Solid Edge part; units mm, degrees
sketch "Sketch1" plane through (0, 0, 0) normal (0, -1, 0) x (1, 0, 0)
  line L0 (22.5, 0) -> (27.5, 0)
  line L1 (27.5, 0) -> (27.5, 5)
  line L2 (27.5, 5) -> (25.5, 5)
  line L3 (25.5, 5) -> (25.5, 10.1495)
  arc A0 (10, 12.9032) -> (25.5, 10.1495) centre (10, -32.0968) cw
  line L4 (0, 12.9032) -> (10, 12.9032)
  line L5 (0, 9.9032) -> (0, 12.9032)
  line L6 (0, 9.9032) -> (10, 9.9032)
  arc A1 (10, 9.9032) -> (22.5, 8) centre (10, -32.0968) cw
  line L7 (22.5, 8) -> (22.5, 0)
  dimension "D1" = 27.5
  dimension "D2" = 27.5
  dimension "D3" = 22.5
revolve "RevolvedProtrusion1" add sketch "Sketch1" angle 360 about axis through (0, 0, 0) along (0, 0, 1)
properties material "Steel"
Here's how the part is built. I have some questions about the finished solid (model axes, mm). A direction names the side the tool comes from. Coordinates: 2 decimals unless noted, no trailing zeros. Order: outer loops, then holes, each group sorted by start corner. A loop starts at its lowest first (then second) coordinate and runs counter-clockwise, first axis right, second up. Notation, with made-up numbers: (81, -37) - (136, -37) arc R11 cw to (136, -19) - close; hole circle Ø1 at (85.25, 43). An arc over 180 degrees is marked (long way). One line per question, with ' | ' between items. Start each with the question number.
1. Which directions (+Z, -Z, +X, -X, +Y, -Y) give clear straight access to the entire face, cutting with the end or side of a thin tool? Please do faces 1 (the flat face through (-23, 0, 0)), 2 (the flat face through (0, 0, 9.903)).
2. I'm going to push flat-ended pins straight in: pin 1 Ø3 at (y, z) = (-16.5, 1.5) entering from +X; pin 2 Ø2 at (x, y) = (21.5, 21.5) entering from +Z; pin 3 Ø16 at (x, y) = (-5, -1.5) entering from -Z; pin 4 Ø2 at (y, z) = (-14.5, 7) entering from -X. Where does each tip first touch, or does it pass through?
3. Please list where these lines run through material, in increasing order: line 1 along X through (y, z) = (0.5, 1.5); line 2 along Y through (x, z) = (0, 5.75); line 3 along Y through (x, z) = (0, 2). Write a range as [from, to].
4. If we mould it in two halves opening along Y, with no side actions, what happens to faces 3 (the flat face through (18.2, -18.2, 5)), 4 (the cylindrical face through (-5.5, -24.9, 7.6)), 5 (the cylindrical face through (-4.878, 21.965, 3.944))? For each: released by +Y, released by -Y, zero draft, split by the parting line, or undercut.
5. If we section it at A-A (z = 2): Write out the boundary of the cut face in (x, y).
Model answer:
1) face 1: -Z, +X, -X, +Y, -Y | face 2: -Z
2) pin 1: stops at x = 23.05 | pin 2: passes through | pin 3: stops at z = 9.78 | pin 4: stops at x = -21.63
3) line 1: x = [-27.5, -22.49], [22.49, 27.5] | line 2: y = [-25.5, -22.5], [22.5, 25.5] | line 3: y = [-27.5, -22.5], [22.5, 27.5]
4) face 3: zero draft | face 4: split by the parting line | face 5: undercut
5) outline: circle Ø55 at (0, 0); hole circle Ø45 at (0, 0)
